Autodesk Fusion 360 part; units mm, degrees
sketch "Esquisse1" plane through (0, 0, 0) normal (0, 1, 0) x (1, 0, 0)
  line L0 (-50, 50) -> (791, 50)
  line L1 (791, 50) -> (791, -544)
  line L2 (791, -544) -> (-50, -544)
  line L3 (-50, -544) -> (-50, 50)
  dimension "d1" = 594
  dimension "d2" = 841
extrude "Extrusion1" add sketch "Esquisse1" along normal blind 20
sketch "Esquisse3" plane through (0, 0, 0) normal (0, 1, 0) x (1, 0, 0)
  line L0 (-50, -544) -> (0, -544)
  line L1 (0, -544) -> (0, 50)
  line L2 (0, 50) -> (-50, 50)
  line L3 (-50, 50) -> (-50, -544)
  line L4 (741, -544) -> (791, -544)
  line L5 (791, -544) -> (791, 50)
  line L6 (791, 50) -> (741, 50)
  line L7 (741, 50) -> (741, -544)
  point P0 (-50, -544)
  point P1 (791, -544)
  point P2 (-25, -247)
  point P3 (766, -247)
  dimension "d7" = 50
  dimension "d8" = 594
  dimension "d9" = 50
  dimension "d10" = 594
extrude "Extrusion2" add sketch "Esquisse3" against normal blind 50
sketch "Esquisse8" plane through (0, 0, 0) normal (1, 0, 0) x (0, 0, -1)
  line L0 (-490, -15) -> (10, -15)
  line L1 (10, -15) -> (10, -50)
  line L2 (10, -50) -> (-490, -50)
  line L3 (-490, -50) -> (-490, -15)
  dimension "d17" = 35
  dimension "d18" = 500
extrude "Extrusion3" cut sketch "Esquisse8" along normal mid plane 1850
fillet "Congé1" radius 25 4 edges at (-50, -15, 544) (-50, -15, -50) (791, -15, 544) (791, -15, -50)
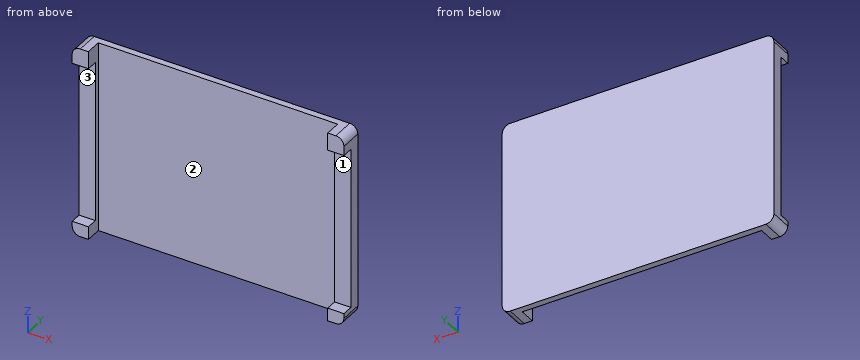
Geometry check sheet. Reference: the model listing, model coordinates, mm. Face numbers are marked on the shaded views. Round coordinates to 2 decimals unless told otherwise and drop trailing zeros. Order: outer loops, then holes, each group sorted by start corner. A loop starts at its lowest first (then second) coordinate and runs counter-clockwise, first axis right, second up. Notation, with made-up numbers: M -8.75,76 L -2.75,76 A22 cw -2.75,114 Z; hole C 5.5,68.25 d9. An arc over 180 degrees is marked long. Write each question's results on one line, items separated by ' | '. Start each with the question number.
1. Material ranges on L1, parallel to Z at x = -11.5, y = -23.5; L2, parallel to X at y = -23, z = -21.5; L3, parallel to Y at x = 362, z = 495, recorded low to high. Write a range as from..to.
2. Go/stop test with flat-tipped pins: P1, Ø4, axis at x = 223, z = 284.5, coming from the -Y side; P2, Ø25, axis at x = -20.5, z = 290, coming from the -Y side. Record where each tip stops, or that it passes through.
3. Cross-section at C-C on x = 214. Record the boundary of the cut face in (y, z).
4. Cross-section at B-B on z = 133. Record the boundary of the cut face in (x, y), plus the area to 3 significant figures.
5. Cross-section at A-A on y = -34. Record the boundary of the cut face in (x, z), plus the area to 3 significant figures.
6. Draft check along Z on the marked faces 1, 2 and 3. Enter one of: pulls with the +Z half, pulls with the -Z half, needs draft (parallel to the pull), parting line crosses it, or undercut.
Resolved:
1) L1: -50..-10, 490..544 | L2: -50..0, 741..791 | L3: 0..20
2) P1: y = 0 | P2: y = -15
3) outline: M 0,-50 L 20,-50 L 20,544 L 0,544 Z
4) outline: M -50,-15 L 0,-15 L 0,0 L 741,0 L 741,-15 L 791,-15 L 791,20 L -50,20 Z | area: 18,300 mm2
5) outline: M -50,-25 A25 ccw -25,-50 L 0,-50 L 0,-10 L -50,-10 Z; M -50,490 L 0,490 L 0,544 L -25,544 A25 ccw -50,519 Z; M 741,-50 L 766,-50 A25 ccw 791,-25 L 791,-10 L 741,-10 Z; M 741,490 L 791,490 L 791,519 A25 ccw 766,544 L 741,544 Z | area: 8,860 mm2
6) face 1: undercut | face 2: needs draft | face 3: undercut
